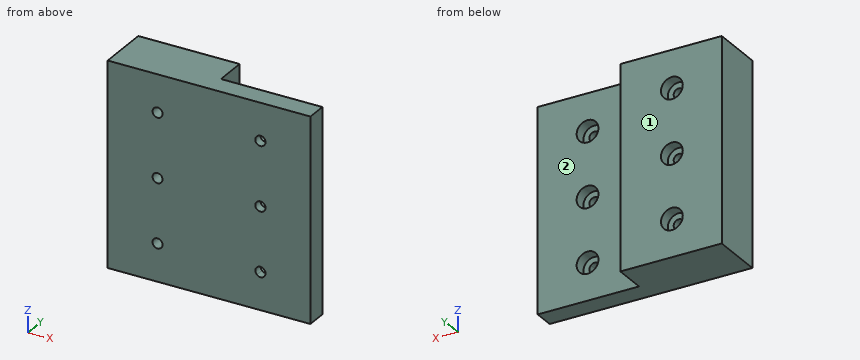
Autodesk Inventor part; units mm, degrees
ref_plane "YZ Plane" through (0, 0, 0) normal (1, 0, 0) x (0, 1, 0)
ref_plane "XZ Plane" through (0, 0, 0) normal (0, 1, 0) x (-1, 0, 0)
ref_plane "XY Plane" through (0, 0, 0) normal (0, 0, 1) x (1, 0, 0)
sketch "Sketch1" plane through (0, 0, 0) normal (0, 1, 0) x (-1, 0, 0)
  line L0 (25, 25) -> (-25, 25)
  line L1 (-25, 25) -> (-25, -25)
  line L2 (-25, -25) -> (25, -25)
  line L3 (25, -25) -> (25, 25)
  line L4 (35, 0) -> (-35, 0)
  line L5 (0, -35) -> (0, 35)
  point P0 (0, 0)
  dimension "d0" = 50
  dimension "d1" = 50
extrude "Extrusion1" add sketch "Sketch1" along normal blind 12.85
sketch "Sketch2" plane through (0, 12.85, 0) normal (0, 1, 0) x (1, 0, 0)
  line L0 (-25, -25) -> (25, -25)
  line L1 (25, -25) -> (25, 25)
  line L2 (0, -25) -> (25, -25)
  line L3 (25, -25) -> (25, 25)
  line L4 (25, 25) -> (0, 25)
  line L5 (0, 25) -> (0, -25)
  point P0 (0, 0)
extrude "Extrusion2" cut sketch "Sketch2" against normal blind 7.85
sketch "Sketch3" plane through (0, 12.85, 0) normal (0, 1, 0) x (1, 0, 0)
  line L0 (-25, -25) -> (25, -25) construction
  line L1 (-12.7037, -25) -> (-12.7037, 25.0391) construction
  line L2 (12.6423, -25) -> (12.6423, 25.0391) construction
  line L3 (-35, 0) -> (35, 0)
  point P0 (0, 0)
  point P1 (-12.7037, -15.7722)
  point P2 (-12.7037, 0.0196)
  point P3 (-12.7037, 15.7722)
  point P4 (12.6423, -15.7722)
  point P5 (12.6423, 0.0196)
  point P6 (12.6423, 15.7722)
hole "Hole1" at (-12.7037, 12.85, 15.7722) at (-12.7037, 12.85, -0.0196) at (-12.7037, 12.85, -15.7722) at (12.6423, 12.85, 15.7722) at (12.6423, 12.85, -0.0196) at (12.6423, 12.85, -15.7722) direction (0, -1, 0) diameter 2.4638 end through all counterbore diameter 5.37 counterbore depth 2.85
sketch "Sketch4" plane through (0, 5, 0) normal (0, 1, 0) x (1, 0, 0)
  point P0 (0, 0)
  point P1 (12.7037, -15.8336)
  point P2 (12.7037, 0)
  point P3 (12.7037, 15.8336)
hole "Hole2" at (12.7037, 5, 0) at (12.7037, 5, -15.8336) at (12.7037, 5, 15.8336) direction (0, -1, 0) diameter 2.4638 end through all counterbore diameter 5.37 counterbore depth 2.85
properties part number "screwbaserecesed"
Geometry check sheet. Reference: the model listing, model coordinates, mm. Face numbers are marked on the shaded views. A direction names the side the tool comes from. Give positions to 0.01 mm unless a question says otherwise; leave off trailing zeros. Order: outer loops, then holes, each group sorted by start corner. A loop starts at its lowest first (then second) coordinate and runs counter-clockwise, first axis right, second up. Notation, with made-up numbers: (38.25, 42.25) - (64.25, 42.25) arc R5 cw to (64.25, 46.25) - close; hole circle Ø9 at (-12.75, 2.25). An arc over 180 degrees is marked (long way). Answer as a JSON object with one key per item and string values.
(1) Tool access check on the marked faces 1 and 2. Record the directions out of +Z, -Z, +X, -X, +Y, -Y that give a thin tool (end or side, any length) a straight path to the whole face; none if there is none.
Report:
{"face 1": "+Z, -Z, +X, -X, +Y", "face 2": "+Z, -Z, +X, +Y"}
(2) Material ranges on line 1 (X direction, y = 7, z = 0); line 2 (Z direction, x = 13, y = 1); line 3 (Z direction, x = 10.5, y = 2.5), recorded low to high.
Report:
{"line 1": "-25 to -13.94, -11.47 to 0", "line 2": "-25 to -17.03, -14.59 to -1.2, 1.2 to 14.59, 17.03 to 25", "line 3": "-25 to -17.37, -14.3 to -1.53, 1.53 to 14.3, 17.37 to 25"}
(3) Cross-section at A-A (z = 0.5). Record the cut outline in (x, y), then the cut area to 3 significant figures.
Report:
{"outline": "(-25, 0) - (-13.82, 0) - (-13.82, 10) - (-15.34, 10) - (-15.34, 12.85) - (-25, 12.85) - close; (-11.59, 0) - (11.53, 0) - (11.53, 2.15) - (10.07, 2.15) - (10.07, 5) - (0, 5) - (0, 12.85) - (-10.07, 12.85) - (-10.07, 10) - (-11.59, 10) - close; (13.83, 0) - (25, 0) - (25, 5) - (15.34, 5) - (15.34, 2.15) - (13.83, 2.15) - close", "area": "389 mm^2"}
(4) Cross-section at B-B (z = 6). Record the cut outline in (x, y).
Report:
{"outline": "(-25, 0) - (25, 0) - (25, 5) - (0, 5) - (0, 12.85) - (-25, 12.85) - close"}
(5) Cross-section at D-D (x = 22.5). Record the cut outline in (y, z).
Report:
{"outline": "(0, -25) - (5, -25) - (5, 25) - (0, 25) - close"}
(6) Depth check by flat-ended pin: pin 1 Ø2 at (x, z) = (-12.7, -0.02) entering from +Y; pin 2 Ø2.5 at (y, z) = (10, -1) entering from +X; pin 3 Ø4.5 at (x, z) = (12.7, 0) entering from +Y; pin 4 Ø4 at (x, z) = (-12.7, -15.77) entering from +Y. Enter the tip coordinate at first touch or a pass-through.
Report:
{"pin 1": "through", "pin 2": "x = 0", "pin 3": "y = 2.15", "pin 4": "y = 10"}
(7) Cross-section at C-C (y = 9). Record the cut outline in (x, z), then the cut area to 3 significant figures.
Report:
{"outline": "(-25, -25) - (0, -25) - (0, 25) - (-25, 25) - close; hole circle Ø2.46 at (-12.7, -15.77); hole circle Ø2.46 at (-12.7, -0.02); hole circle Ø2.46 at (-12.7, 15.77)", "area": "1,240 mm^2"}
